The listing builds one solid part. Answer for the finished solid, in the listing's coordinates (mm). A direction names the side the tool comes from. Coordinates: 2 decimals unless noted, no trailing zeros. Loops run counter-clockwise (first coordinate to the right, second up) from the corner with the lowest first, then second, coordinate; pieces in that order, holes last. Notation, with made-up numbers: (72, 77.5) - (88, 77.5) arc R19 ccw to (88, 100.5) - close; hole circle Ø11 at (58, 83.5). An arc over 180 degrees is marked (long way). Write each question's results on one line, items separated by ' | '. Start each with the question number.
(1) For faces 1 (the cylindrical face through (-4.496, -15.802, 25.497)), 2 (the flat face through (-5, -27, 0)), 3 (the flat face through (-6, -25, 0)), determine the directions among +Z, -Z, +X, -X, +Y, -Y from which every point of the face is accessible in a straight line to the end or side of a thin tool.
(2) Given pin 1 Ø5 at (x, z) = (18, -10) entering from +Y; pin 2 Ø10 at (x, y) = (-12, -7) entering from +Z; pin 3 Ø8 at (x, y) = (16, -6) entering from -Z, each flat-ended and moving along its own axis, determine where each tip first touches the part or whether it passes through.
(3) Consider line 1 (Y direction, x = 0, z = 26); line 2 (Z direction, x = 0, y = -9); line 3 (Z direction, x = -18, y = -15.5). Determine where each line is inside the solid, lowest interval first. Write a range as from..to.
(4) Find section D-D on y = -9. Determine the outline of the cut face in (x, z).
(5) Determine the mould class of faces 4 (the flat face through (-6, 0, 23)), 5 (the cylindrical face through (-4.496, -15.802, -25.497)), 6 (the flat face through (6, -30, 0)), 7 (the cylindrical face through (4.1, -27.46, 15.64)) for opening direction Y: released by +Y, released by -Y, zero draft, split by the parting line, or undercut.
(6) Find section B-B on x = 0. Determine the outline of the cut face in (y, z).
(7) Find section A-A on z = 0. Determine the outline of the cut face in (x, y).
(8) Find section C-C on y = -16. Determine the outline of the cut face in (x, z), then the cut area to 3 significant figures.
from build123d import *

# Parameters (mm, degrees)
F0_R          = 28
F0_R_2        = 23.5
F1_DEPTH      = 25
F2_R          = 28
F3_DEPTH      = 5
F5_R          = 4.5
F6_DEPTH      = 50
F6_DEPTH_BACK = 50


with BuildPart() as f1:
    # F0 (on Front) → F1 (new body)
    with BuildSketch(Plane.XZ):
        Circle(F0_R)
        Circle(F0_R_2, mode=Mode.SUBTRACT)
    extrude(amount=F1_DEPTH)

    # F2 (on face) → F3 (join)
    with BuildSketch(Plane.XZ.offset(25)):
        Circle(F2_R)
        with BuildLine():
            Line((-5, -13.5), (-5, 13.5))
            ThreePointArc((-5, 13.5), (-4.12132, 15.62132), (-2, 16.5))
            Line((-2, 16.5), (2, 16.5))
            ThreePointArc((2, 16.5), (4.12132, 15.62132), (5, 13.5))
            Line((5, 13.5), (5, -13.5))
            ThreePointArc((5, -13.5), (4.12132, -15.62132), (2, -16.5))
            Line((2, -16.5), (-2, -16.5))
            ThreePointArc((-2, -16.5), (-4.12132, -15.62132), (-5, -13.5))
        make_face(mode=Mode.SUBTRACT)
    extrude(amount=F3_DEPTH)

    # F5 (on Top) → F6 (cut, two sides)
    with BuildSketch(Plane.XY) as f6_sk:
        with Locations((0, -16)):
            Circle(F5_R)
    extrude(amount=F6_DEPTH, mode=Mode.SUBTRACT)
    extrude(f6_sk.sketch, amount=-F6_DEPTH_BACK, mode=Mode.SUBTRACT)


solid = f1.part
Values:
1) face 1: +Z, -Z | face 2: +Y, -Y | face 3: +Y
2) pin 1: stops at y = -25 | pin 2: stops at z = 27.11 | pin 3: stops at z = -25.3
3) line 1: y = -30..-20.5, -11.5..0 | line 2: z = -28..-23.5, 23.5..28 | line 3: z = -21.45..-15.11, 15.11..21.45
4) outline: circle Ø56 at (0, 0); hole circle Ø47 at (0, 0)
5) face 4: released by +Y | face 5: undercut | face 6: released by -Y | face 7: zero draft
6) outline: (-30, -28) - (-20.5, -28) - (-20.5, -23.5) - (-25, -23.5) - (-25, -16.5) - (-30, -16.5) - close; (-30, 16.5) - (-25, 16.5) - (-25, 23.5) - (-20.5, 23.5) - (-20.5, 28) - (-30, 28) - close; (-11.5, -28) - (0, -28) - (0, -23.5) - (-11.5, -23.5) - close; (-11.5, 23.5) - (0, 23.5) - (0, 28) - (-11.5, 28) - close
7) outline: (-28, -30) - (-5, -30) - (-5, -25) - (-23.5, -25) - (-23.5, 0) - (-28, 0) - close; (5, -30) - (28, -30) - (28, 0) - (23.5, 0) - (23.5, -25) - (5, -25) - close
8) outline: (-4.5, -27.64) - (-4.5, -23.07) arc R23.5 cw to (-4.5, 23.07) - (-4.5, 27.64) arc R28 ccw to start; (4.5, -27.64) arc R28 ccw to (4.5, 27.64) - (4.5, 23.07) arc R23.5 cw to (4.5, -23.07) - close | area: 647 mm²
